The listing builds one solid part. Answer for the finished solid, in the listing's coordinates (mm). Face numbers are marked on the shaded views. A direction names the side the tool comes from. Give positions to 0.01 mm unless a question says otherwise; leave off trailing zeros. Loops run counter-clockwise (first coordinate to the right, second up) from the corner with the lowest first, then second, coordinate; pieces in that order, holes last. Notation, with made-up numbers: M 82.25,67 L 140.25,67 A23 ccw 140.25,99 Z; hole C 30.25,56.25 d5. An arc over 180 degrees is marked long. Return JSON: item names as keys, results as strings.
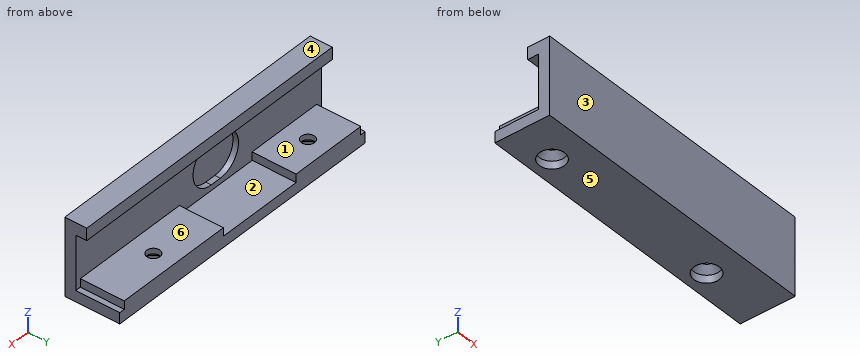
from build123d import *

# Parameters (mm, degrees)
SKETCH2_W                           = 68.58
SKETCH2_H                           = 17.78
BOSS_EXTRUDE1_DEPTH                 = 2.54
SKETCH3_W                           = 68.58
SKETCH3_H                           = 2.54
BOSS_EXTRUDE2_DEPTH                 = 2.54
BOSS_EXTRUDE3_DEPTH                 = 10.16
SKETCH5_R                           = 1.524
CUT_EXTRUDE1_DEPTH                  = 72.009355898
CUT_EXTRUDE2_START                  = -3.81
SKETCH6_R                           = 2.921
CUT_EXTRUDE2_DEPTH                  = 68.199355898
CHAMFER1_SIZE                       = 2.54
CUT_EXTRUDE3_DEPTH                  = 1.27
SKETCH8_W                           = 68.58
SKETCH8_H                           = 2.54
EXTRA_WIDTH_FOR_MIRRORED_PART_DEPTH = 0.254


with BuildPart() as part:
    # Sketch2 → Boss-Extrude1 (new body)
    with BuildSketch(Plane(origin=(0, 0, 0), x_dir=(1, 0, 0), z_dir=(0, 1, 0))):
        with Locations((34.29, -8.89)):
            Rectangle(SKETCH2_W, SKETCH2_H)
    extrude(amount=BOSS_EXTRUDE1_DEPTH)

    # Sketch3 → Boss-Extrude2 (add)
    with BuildSketch(Plane(origin=(0, 2.54, 0), x_dir=(1, 0, 0), z_dir=(0, 1, 0))):
        with Locations((34.29, -16.51)):
            Rectangle(SKETCH3_W, SKETCH3_H)
    extrude(amount=BOSS_EXTRUDE2_DEPTH)

    # Sketch4 → Boss-Extrude3 (add)
    with BuildSketch(Plane(origin=(0, 2.54, 0), x_dir=(1, 0, 0), z_dir=(0, 1, 0))):
        Polygon((0, 0), (68.58, 0), (68.58, -2.54), (67.31, -2.54), (67.31, -4.445), (39.624, -4.445), (39.624, -2.54), (19.304, -2.54), (19.304, -4.445), (1.27, -4.445), (1.27, -2.54), (0, -2.54), align=None)
    extrude(amount=BOSS_EXTRUDE3_DEPTH)

    # Sketch5 → Cut-Extrude1 (cut, through all)
    with BuildSketch(Plane.XY.offset(4.445)):
        with Locations((10.16, 7.874)):
            Circle(SKETCH5_R)
        with Locations((53.34, 7.874)):
            Circle(SKETCH5_R)
    extrude(amount=-CUT_EXTRUDE1_DEPTH, mode=Mode.SUBTRACT)

    # Sketch6 → Cut-Extrude2 (cut, through all)
    with BuildSketch(Plane.XY.offset(4.445).offset(CUT_EXTRUDE2_START)):
        with Locations((10.16, 7.874)):
            Circle(SKETCH6_R)
        with Locations((53.34, 7.874)):
            Circle(SKETCH6_R)
    extrude(amount=-CUT_EXTRUDE2_DEPTH, mode=Mode.SUBTRACT)

    # Chamfer1
    # the kernel refuses this chamfer: 2.54 mm, written as the material it takes off along each edge
    with BuildSketch(Plane(origin=(53.34, 7.874, 0.635), x_dir=(1, 0, 0), z_dir=(0, -1, 0))) as chamfer1_piece_1_section:
        Polygon((1.524 + CHAMFER1_SIZE, 0), (1.524, CHAMFER1_SIZE), (1.524, 0), align=None)
    chamfer1_piece_1 = revolve(axis=Axis((53.34, 7.874, 0.635), (0, 0, 1)), mode=Mode.PRIVATE)
    chamfer1_piece_1 = chamfer1_piece_1 & Plane(origin=(53.34, 7.874, 2.488878995), x_dir=(1, 0, 0), z_dir=(0, 0, 1)) * Cylinder(2.921, 17, mode=Mode.PRIVATE)
    add(chamfer1_piece_1, mode=Mode.SUBTRACT)
    with BuildSketch(Plane(origin=(10.16, 7.874, 0.635), x_dir=(1, 0, 0), z_dir=(0, -1, 0))) as chamfer1_piece_2_section:
        Polygon((1.524 + CHAMFER1_SIZE, 0), (1.524, CHAMFER1_SIZE), (1.524, 0), align=None)
    chamfer1_piece_2 = revolve(axis=Axis((10.16, 7.874, 0.635), (0, 0, 1)), mode=Mode.PRIVATE)
    chamfer1_piece_2 = chamfer1_piece_2 & Plane(origin=(10.16, 7.874, 2.488878995), x_dir=(1, 0, 0), z_dir=(0, 0, 1)) * Cylinder(2.921, 17, mode=Mode.PRIVATE)
    add(chamfer1_piece_2, mode=Mode.SUBTRACT)

    # Sketch7 → Cut-Extrude3 (cut)
    with BuildSketch(Plane(origin=(0, 2.54, 0), x_dir=(1, 0, 0), z_dir=(0, 1, 0))):
        with BuildLine():
            Line((28.194, -3.81), (30.734, -3.81))
            ThreePointArc((30.734, -3.81), (35.814, -8.89), (30.734, -13.97))
            Line((30.734, -13.97), (28.194, -13.97))
            ThreePointArc((28.194, -13.97), (23.114, -8.89), (28.194, -3.81))
        make_face()
    extrude(amount=-CUT_EXTRUDE3_DEPTH, mode=Mode.SUBTRACT)

    # Sketch8 → Extra_width_for_mirrored_part (add)
    with BuildSketch(Plane(origin=(0, 0, 15.24), x_dir=(-1, 0, 0), z_dir=(0, 0, -1))):
        with Locations((-34.29, 3.81)):
            Rectangle(SKETCH8_W, SKETCH8_H)
    extrude(amount=EXTRA_WIDTH_FOR_MIRRORED_PART_DEPTH)


solid = part.part
(1) The part is cut by section B-B (y = 3.5). Determine the outline of the cut face in (x, z) (3 decimals).
Values follow:
{"outline": "M 0,0 L 68.58,0 L 68.58,2.54 L 67.31,2.54 L 67.31,4.445 L 39.624,4.445 L 39.624,2.54 L 19.304,2.54 L 19.304,4.445 L 1.27,4.445 L 1.27,2.54 L 0,2.54 Z; M 0,14.986 L 68.58,14.986 L 68.58,17.78 L 0,17.78 Z"}
(2) The part is cut by section C-C (z = 8.89). Determine the outline of the cut face in (x, y), and give its area (3 significant figures).
Values follow:
{"outline": "M 0,0 L 68.58,0 L 68.58,2.54 L 35.81,2.54 L 35.81,1.27 L 23.11,1.27 L 23.11,2.54 L 0,2.54 Z", "area": "158 mm²"}
(3) A tool of negligible diameter and unlimited length cuts with its end or side. For the marked faces 1 and 2, from which of +Z, -Z, +X, -X, +Y, -Y can it reach the whole face along a straight path? Write none if from no direction.
Values follow:
{"face 1": "+X, -X, +Y", "face 2": "+Y"}
(4) Determine the mould class of the marked faces 3, 4, 5 and 6 for opening direction Z: released by +Z, released by -Z, zero draft, split by the parting line, or undercut.
Values follow:
{"face 3": "zero draft", "face 4": "released by +Z", "face 5": "released by -Z", "face 6": "undercut"}
(5) Straight lines are drawn through the part: line 1 along Z through (x, y) = (28.5, 4.25); line 2 along Y through (x, z) = (53.34, 3.65); line 3 along Z through (x, y) = (7.5, 9.25) (3 decimals). For each, find the intervals that lie inside material, in ascending order.
Values follow:
{"line 1": "0 to 2.54, 14.99 to 17.78", "line 2": "0 to 6.35, 9.4 to 12.7", "line 3": "0 to 4.445"}
(6) The part is cut by section D-D (y = 11.5). Determine the outline of the cut face in (x, z) (3 decimals), and give its area (3 significant figures).
Values follow:
{"outline": "M 0,0 L 68.58,0 L 68.58,2.54 L 67.31,2.54 L 67.31,4.445 L 39.624,4.445 L 39.624,2.54 L 19.304,2.54 L 19.304,4.445 L 1.27,4.445 L 1.27,2.54 L 0,2.54 Z", "area": "261 mm²"}
(7) Given pin 1 (1.3 mm diameter, centred on x = 17.5, y = 4.5, fed in from -Z); pin 2 (2 mm diameter, centred on y = 8, z = 5, fed in from +X); pin 3 (1.5 mm diameter, centred on y = 8, z = 3.5, fed in from -X); pin 4 (1 mm diameter, centred on x = 68, y = 6, fed in from +Z), each flat-ended and moving along its own axis, determine where each tip first touches the part or whether it passes through.
Values follow:
{"pin 1": "z = 0", "pin 2": "x = 67.31", "pin 3": "x = 1.27", "pin 4": "z = 2.54"}
(8) The part is cut by section A-A (x = 53.34). Determine the outline of the cut face in (y, z) (3 decimals), and give its area (3 significant figures).
Values follow:
{"outline": "M 0,0 L 4.953,0 L 4.953,1.778 L 6.35,3.175 L 6.35,4.445 L 2.54,4.445 L 2.54,14.986 L 5.08,14.986 L 5.08,17.78 L 0,17.78 Z; M 9.398,3.175 L 10.795,1.778 L 10.795,0 L 12.7,0 L 12.7,4.445 L 9.398,4.445 Z", "area": "77.0 mm²"}
